from build123d import *

# Parameters (mm, degrees)
SKETCH_1_R          = 2.5
EXTRUDE_1_DEPTH     = 950
SKETCH_2_W          = 109.948268043
SKETCH_2_H          = 29.443949836
CUT_EXTRUDE_1_DEPTH = 725.86


with BuildPart() as part:
    # 草图1 → 凸台-拉伸1 (new body)
    with BuildSketch(Plane.XY):
        with BuildLine():
            Line((-8.2, -3.1), (-10, -3.1))
            Line((-10, -3.1), (-10, -8.5))
            ThreePointArc((-10, -8.5), (-9.560660172, -9.560660172), (-8.5, -10))
            Line((-8.5, -10), (-3.1, -10))
            Line((-3.1, -10), (-3.1, -8.2))
            Line((-3.1, -8.2), (-5.5, -8.2))
            Line((-5.5, -8.2), (-5.5, -6.397050155))
            Line((-5.5, -6.397050155), (-2.202949845, -3.1))
            Line((-2.202949845, -3.1), (2.202949845, -3.1))
            Line((2.202949845, -3.1), (5.5, -6.397050155))
            Line((5.5, -6.397050155), (5.5, -8.2))
            Line((5.5, -8.2), (3.1, -8.2))
            Line((3.1, -8.2), (3.1, -10))
            Line((3.1, -10), (8.5, -10))
            ThreePointArc((8.5, -10), (9.560660172, -9.560660172), (10, -8.5))
            Line((10, -8.5), (10, -3.1))
            Line((10, -3.1), (8.2, -3.1))
            Line((8.2, -3.1), (8.2, -5.5))
            Line((8.2, -5.5), (6.397050155, -5.5))
            Line((6.397050155, -5.5), (3.05412702, -2.157076865))
            Line((3.05412702, -2.157076865), (3.05412702, 2.157076865))
            Line((3.05412702, 2.157076865), (6.397050155, 5.5))
            Line((6.397050155, 5.5), (8.2, 5.5))
            Line((8.2, 5.5), (8.2, 3.1))
            Line((8.2, 3.1), (10, 3.1))
            Line((10, 3.1), (10, 8.5))
            ThreePointArc((10, 8.5), (9.560660172, 9.560660172), (8.5, 10))
            Line((8.5, 10), (3.1, 10))
            Line((3.1, 10), (3.1, 8.2))
            Line((3.1, 8.2), (5.5, 8.2))
            Line((5.5, 8.2), (5.5, 6.397050155))
            Line((5.5, 6.397050155), (2.202949845, 3.1))
            Line((2.202949845, 3.1), (-2.202949845, 3.1))
            Line((-2.202949845, 3.1), (-5.5, 6.397050155))
            Line((-5.5, 6.397050155), (-5.5, 8.2))
            Line((-5.5, 8.2), (-3.1, 8.2))
            Line((-3.1, 8.2), (-3.1, 10))
            Line((-3.1, 10), (-8.5, 10))
            ThreePointArc((-8.5, 10), (-9.560660172, 9.560660172), (-10, 8.5))
            Line((-10, 8.5), (-10, 3.1))
            Line((-10, 3.1), (-8.2, 3.1))
            Line((-8.2, 3.1), (-8.2, 5.5))
            Line((-8.2, 5.5), (-6.397050155, 5.5))
            Line((-6.397050155, 5.5), (-3.05412702, 2.157076865))
            Line((-3.05412702, 2.157076865), (-3.05412702, -2.157076865))
            Line((-3.05412702, -2.157076865), (-6.397050155, -5.5))
            Line((-6.397050155, -5.5), (-8.2, -5.5))
            Line((-8.2, -5.5), (-8.2, -3.1))
        make_face()
        with Locations(Location((0, 0, 0), (0, 0, 180))):
            Circle(SKETCH_1_R, mode=Mode.SUBTRACT)
    extrude(amount=EXTRUDE_1_DEPTH)

    # 草图2 → 切除-拉伸1 (cut)
    with BuildSketch(Plane.XY.offset(950)):
        with Locations((27.511129311, -2.182282155)):
            Rectangle(SKETCH_2_W, SKETCH_2_H)
    extrude(amount=-CUT_EXTRUDE_1_DEPTH, mode=Mode.SUBTRACT)


solid = part.part
Verification items for the finished model (mm, model axes). A direction names the side the tool comes from. Round coordinates to 2 decimals unless told otherwise and drop trailing zeros. Write each loop counter-clockwise with the first axis right and the second up, starting at its lowest first coordinate (ties: lowest second). Pieces come first, ordered by that corner, then holes.
(1) Mould release check, pull along Y, two halves, no side actions. Record for faces 1 (the cylindrical face through (2.5, -0.1, 110.5)), 2 (the flat face through (-6, 10, 111)), 3 (the flat face through (3.054, 0, 111)), 4 (the flat face through (6, -10, 111)): pulls with the +Y half, pulls with the -Y half, needs draft (parallel to the pull), parting line crosses it, or undercut.
Returned:
face 1: undercut
face 2: pulls with the +Y half
face 3: undercut
face 4: pulls with the -Y half
(2) Section check A-A (y = 0). Enter the section's corners in (x, z).
Returned:
outline: (-3.05, 0) - (-2.5, 0) - (-2.5, 224.14) - (-3.05, 224.14) - close; (2.5, 0) - (3.05, 0) - (3.05, 224.14) - (2.5, 224.14) - close
(3) Depth check by flat-ended pin: pin 1 Ø10 at (y, z) = (1, 141.5) entering from +X; pin 2 Ø3.5 at (x, z) = (0, 66) entering from -Y; pin 3 Ø2 at (x, y) = (-6, 2) entering from +Z; pin 4 Ø2 at (y, z) = (-0.5, 91.5) entering from +X. Enter the tip coordinate at first touch or a pass-through.
Returned:
pin 1: stops at x = 10
pin 2: stops at y = -3.1
pin 3: passes through
pin 4: stops at x = 3.05
(4) Access from +Z, -Z, +X, -X, +Y, -Y to the whole of each face (thin tool, end or side, straight path). Record for faces 5 (the flat face through (0, 3.1, 111)), 6 (the flat face through (-3.054, 0, 111)), 7 (the flat face through (0, -3.1, 111)).
Returned:
face 5: +Z, -Z, +Y
face 6: +Z, -Z, -X
face 7: +Z, -Z, -Y
(5) Material ranges on line 1 (Y direction, x = 3.5, z = 211); line 2 (Y direction, x = 0, z = 159); line 3 (X direction, y = 4, z = 211), recorded low to high.
Returned:
line 1: y = -10 to -8.2, -4.4 to -2.6, 2.6 to 4.4, 8.2 to 10
line 2: y = -3.1 to -2.5, 2.5 to 3.1
line 3: x = -10 to -8.2, -4.9 to -3.1, 3.1 to 4.9, 8.2 to 10
(6) Section check B-B (x = 0). Enter the section's corners in (y, z), plus the area to 3 significant figures.
Returned:
outline: (-3.1, 0) - (-2.5, 0) - (-2.5, 224.14) - (-3.1, 224.14) - close; (2.5, 0) - (3.1, 0) - (3.1, 224.14) - (2.5, 224.14) - close
area: 269 mm2
